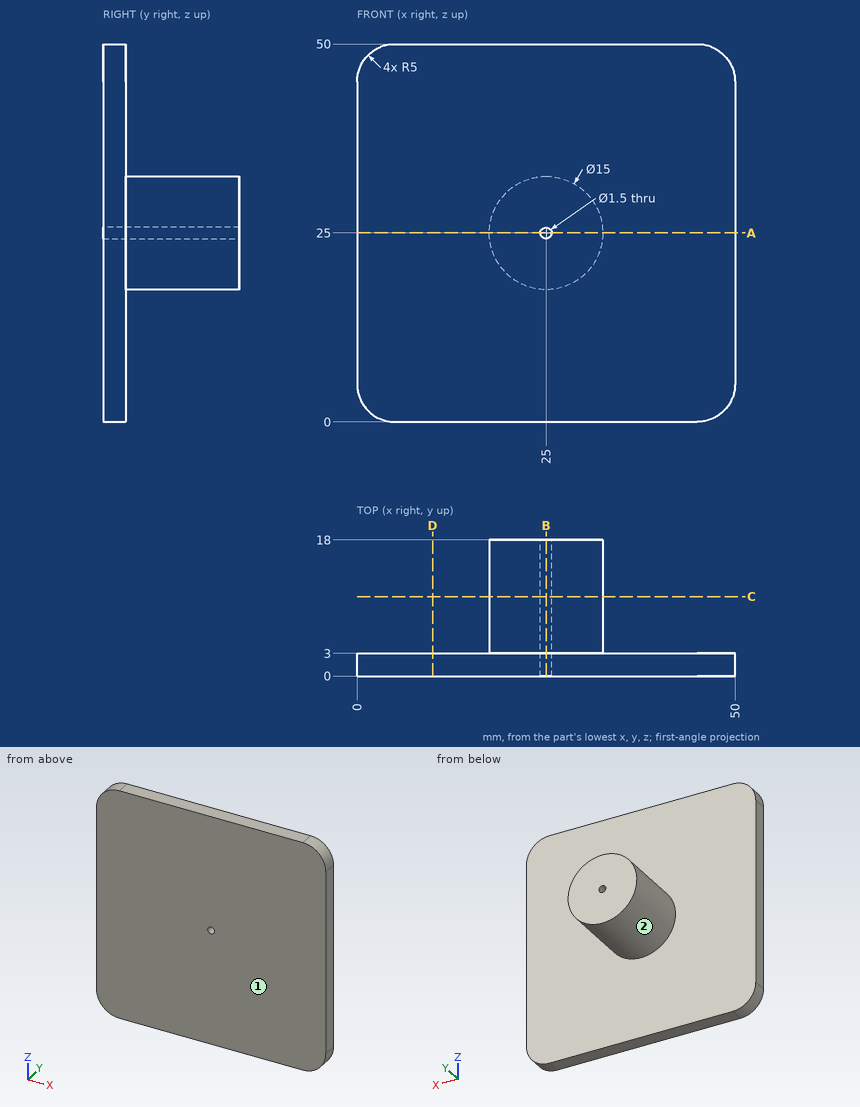
Can you work these out from the drawing? Everything is in mm from the part's minimum corner. A direction names the side the tool comes from. Round coordinates to 2 decimals unless told otherwise and drop trailing zeros. Order: outer loops, then holes, each group sorted by start corner. A loop starts at its lowest first (then second) coordinate and runs counter-clockwise, first axis right, second up. Notation, with made-up numbers: M -18.75,54.25 L -11.75,54.25 A32 ccw -11.75,84.25 Z; hole C 21,30 d3. An arc over 180 degrees is marked long. Answer as CSV lines item,"result".
Item 1: Imagine slicing it at C-C on y = 10.5. List the corners of the cut face in (x, z) for me, and give its area (3 significant figures).
From the geometry:
outline,"C 25,25 d15; hole C 25,25 d1.5"
area,"175 mm2"
Item 2: Imagine slicing it at D-D on x = 10. List the corners of the cut face in (y, z) for me.
From the geometry:
outline,"M 0,0 L 3,0 L 3,50 L 0,50 Z"
Item 3: Imagine slicing it at A-A on z = 25. List the corners of the cut face in (x, y) for me, and give its area (3 significant figures).
From the geometry:
outline,"M 0,0 L 24.25,0 L 24.25,18 L 17.5,18 L 17.5,3 L 0,3 Z; M 25.75,0 L 50,0 L 50,3 L 32.5,3 L 32.5,18 L 25.75,18 Z"
area,"348 mm2"
Item 4: Imagine slicing it at B-B on x = 25. List the corners of the cut face in (y, z) for me.
From the geometry:
outline,"M 0,0 L 3,0 L 3,17.5 L 18,17.5 L 18,24.25 L 0,24.25 Z; M 0,25.75 L 18,25.75 L 18,32.5 L 3,32.5 L 3,50 L 0,50 Z"
Item 5: For pin 1 (10 mm diameter, centred on x = 33, y = 13.5, fed in from +Z), with a flat end and sliding along its axis, tell me the tip position at first contact or that it passes through.
From the geometry:
pin 1,"z = 31.87"
Item 6: Please list where these lines run through material, in increasing order: L1, parallel to X at y = 5, z = 25; L2, parallel to Y at x = 4, z = 41; L3, parallel to X at y = 11.5, z = 25.5. Write a range as [from, to].
From the geometry:
L1,"[17.5, 24.25], [25.75, 32.5]"
L2,"[0, 3]"
L3,"[17.52, 24.44], [25.56, 32.48]"
Item 7: Which directions (+Z, -Z, +X, -X, +Y, -Y) give clear straight access to the entire face, cutting with the end or side of a thin tool? Please do the marked faces 1 and 2.
From the geometry:
face 1,"+Z, -Z, +X, -X, -Y"
face 2,"+Y"
